Check sheet for the modelled part. Datum: model origin and axes. Units: mm. A direction names the side the tool comes from. Round coordinates to 2 decimals unless told otherwise and drop trailing zeros. Order: outer loops, then holes, each group sorted by start corner. A loop starts at its lowest first (then second) coordinate and runs counter-clockwise, first axis right, second up.
Q1. Scan lines: probe 1 along Z at (x, y) = (0, 1.7); probe 2 along Y at (x, z) = (-13.5, -10.5); probe 3 along Y at (x, z) = (-14, -7). Record each from-to range of solid material in increasing order.
Q2. Mould release check, pull along X, two halves, no side actions. Record for faces 4 (the flat face through (6, -22, 0)), 5 (the cylindrical face through (-14.642, 1.521, -7.59)), 6 (the flat face through (9, -16, 0)): +X half, -X half, draft (parallel to the pull), parting line (faces both ways), or undercut.
Q3. Cross-section at D-D on y = -17. Record the cut outline in (x, z).
Q4. Depth check by flat-ended pin: P1, Ø4, axis at x = 11, z = 14, coming from the -Y side; P2, Ø10, axis at x = -7.5, y = 3.5, coming from the -Z side; P3, Ø5, axis at y = -14.5, z = -0.5, coming from the +X side. Enter the tip coordinate at first touch or a pass-through.
Q5. Set-up check for faces 1 (the cylindrical face through (14.6, 10.6, 11.2)), 2 (the flat face through (10.3, -6.5, 0.1)), 3 (the cylindrical face through (-14.2, 36.8, -10.9)): record each of +Z, -Z, +X, -X, +Y, -Y from which the full face is reachable in a straight line by a thin tool's end or side.
Q6. Cross-section at C-C on y = 47.5. Record the cut outline in (x, z), then the cut area to 3 significant figures.
Autodesk Inventor part; units mm, degrees
ref_plane "YZ Plane" through (0, 0, 0) normal (1, 0, 0) x (0, 1, 0)
ref_plane "XZ Plane" through (0, 0, 0) normal (0, 1, 0) x (-1, 0, 0)
ref_plane "XY Plane" through (0, 0, 0) normal (0, 0, 1) x (1, 0, 0)
sketch "Sketch1" plane through (0, 0, 0) normal (0, 1, 0) x (-1, 0, 0)
  circle A0 centre (0, 0) radius 18.4
  dimension "d0" = 36.8
extrude "Extrusion1" add sketch "Sketch1" along normal blind 22
sketch "Sketch2" plane through (0, 22, 0) normal (0, 1, 0) x (1, 0, 0)
  circle A0 centre (0, 0) radius 18.4
  circle A1 centre (0, 0) radius 17.9
  dimension "d3" = 35.8
extrude "Extrusion2" add sketch "Sketch2" along normal blind 30 contours A1
fillet "Fillet1" radius 0.5 1 edges at (18.4, 22, 0)
sketch "Sketch3" plane through (0, 0, 0) normal (0, -1, 0) x (1, 0, 0)
  circle A0 centre (0, 0) radius 18.4
  line L0 (0, 0) -> (7, 0)
  circle A1 centre (7, 0) radius 6
  dimension "d7" = 7
  dimension "d8" = 12
extrude "Extrusion3" add sketch "Sketch3" along normal blind 6.5 contours A1
sketch "Sketch4" plane through (7, -6.5, 0) normal (0, -1, 0) x (1, 0, 0)
  circle A0 centre (0, 0) radius 6
  circle A1 centre (0, 0) radius 3
  point P0 (-7, 0)
  dimension "d11" = 6
extrude "Extrusion4" add sketch "Sketch4" along normal blind 3.5 contours A1
sketch "Sketch5" plane through (7, -10, 0) normal (0, -1, 0) x (1, 0, 0)
  circle A0 centre (0, 0) radius 3
  point P0 (-7, 0)
extrude "Extrusion5" add sketch "Sketch5" along normal blind 12
chamfer "Chamfer1" distance 1 angle 45 1 edges at (1, -6.5, 0)
sketch "Sketch6" plane through (7, -22, 0) normal (0, -1, 0) x (1, 0, 0)
  circle A0 centre (0, 0) radius 3
  line L0 (3, 0) -> (2.4, 0)
  line L1 (3.4, -3) -> (2, -3)
  line L2 (2, -3) -> (2, 3)
  line L3 (2, 3) -> (3.4, 3)
  line L4 (3.4, 3) -> (3.4, -3)
  line L5 (3.4, -3) -> (2, 3) construction
  line L6 (2, -3) -> (3.4, 3) construction
  point P0 (-7, 0)
  point P1 (2.7, 0)
  dimension "d19" = 0.6
extrude "Extrusion6" cut sketch "Sketch6" against normal blind 12 contours A0 L2 | A0 L2 L3 L4 L1 picked at (2.1409, -0.5898)
sketch "Sketch7" plane through (0, 0, 0) normal (0, -1, 0) x (1, 0, 0)
  circle A0 centre (0, 0) radius 18.4
  circle A1 centre (0, 0) radius 15.5
  circle A2 centre (0, 15.5) radius 1.2
  circle A3 centre (0, -15.5) radius 1.2
  circle A4 centre (-13.4234, -7.75) radius 1.2
  circle A5 centre (13.4234, -7.75) radius 1.2
  circle A6 centre (-13.4234, 7.75) radius 1.2
  circle A7 centre (13.4234, 7.75) radius 1.2
  dimension "d22" = 31
  dimension "d23" = 2.4
  dimension "d24" = 2.4
  dimension "d28" = 2.4
  dimension "d29" = 2.4
  dimension "d32" = 2.4
  dimension "d33" = 15.5
  dimension "d34" = 2.4
hole "Hole1" at (13.4234, 0, 7.75) at (13.4234, 0, -7.75) at (0, 0, 15.5) at (-13.4234, 0, 7.75) at (-13.4234, 0, -7.75) at (0, 0, -15.5) direction (0, 1, 0) diameter 2.459 depth 3
properties part number "DC_motor_with_encoder"
Results found:
1. probe 1: z = -18.4 to -16.73, -14.27 to 14.27, 16.73 to 18.4
1. probe 2: y = 0 to 52
1. probe 3: y = 3 to 52
2. face 4: draft
2. face 5: undercut
2. face 6: +X half
3. outline: (9, -2.24) - (9, 2.24) arc R3 ccw (long way) to start
4. P1: stops at y = 0
4. P2: stops at z = -18.23
4. P3: stops at x = 9
5. face 1: +Y, -Y
5. face 2: -Y
5. face 3: +Y
6. outline: circle Ø35.8 at (0, 0)
6. area: 1,010 mm2
